Work out the finished part from the listing and answer in its coordinate system (mm). A direction names the side the tool comes from. Round coordinates to 2 decimals unless told otherwise and drop trailing zeros. Loops run counter-clockwise (first coordinate to the right, second up) from the corner with the lowest first, then second, coordinate; pieces in that order, holes last. Notation, with made-up numbers: M 30.25,80 L 35.25,80 A22 cw 35.25,112 Z; hole C 81,-29 d6. An arc over 180 degrees is marked long. One line per item, written item: value.
```python
from build123d import *

# Parameters (mm, degrees)
F0_W     = 4.318
F0_H     = 1.4593527386
F1_DEPTH = 2


with BuildPart() as f1:
    # F0 (on Top) → F1 (new body)
    with BuildSketch(Plane.XY):
        with Locations((4.9730502656, -0.8943877724)):
            Rectangle(F0_W, F0_H)
        with BuildLine():
            Line((7.1320502656, -1.6240641417), (2.8140502656, -1.6240641417))
            Line((2.8140502656, -1.6240641417), (2.8140502656, -0.1647114031))
            Line((2.8140502656, -0.1647114031), (2.6522759268, -0.1647114031))
            Line((2.6522759268, -0.1647114031), (2.6522759268, -19.4612857813))
            Line((2.6522759268, -19.4612857813), (4.8948850305, -19.4612857813))
            Line((4.8948850305, -19.4612857813), (4.8948850305, -11.436884092))
            Line((4.8948850305, -11.436884092), (8.9239793524, -11.436884092))
            Line((8.9239793524, -11.436884092), (13.5950258095, -19.4612857813))
            Line((13.5950258095, -19.4612857813), (16.2473017363, -19.4612857813))
            Line((16.2473017363, -19.4612857813), (11.0061004223, -10.7907085875))
            add(Edge.make_bspline(
                [(14.8873768184, -5.6170811825), (14.8873768184, -9.4434537776), (11.0061004223, -10.7907085875)],
                knots=[0, 0, 0, 1, 1, 1], degree=2))
            add(Edge.make_bspline(
                [(13.1916940404, -1.524636321), (14.8873768184, -2.8845612389), (14.8873768184, -5.6170811825)],
                knots=[0, 0, 0, 1, 1, 1], degree=2))
            add(Edge.make_bspline(
                [(11.4500502656, -0.6254353556), (12.4829894147, -0.9562605066), (13.1916940404, -1.524636321)],
                knots=[0.5820535333, 0.5820535333, 0.5820535333, 1, 1, 1], degree=2))
            Line((11.4500502656, -0.6254353556), (11.4500502656, -1.6240641417))
            Line((11.4500502656, -1.6240641417), (7.1320502656, -1.6240641417))
        make_face()
        with BuildLine():
            Line((7.9737212576, -9.5110276865), (4.8948850305, -9.5110276865))
            Line((4.8948850305, -9.5110276865), (4.8948850305, -2.1328015016))
            Line((4.8948850305, -2.1328015016), (7.8132332238, -2.1328015016))
            add(Edge.make_bspline(
                [(11.436884092, -2.9774753637), (10.3092444862, -2.1328015016), (7.8132332238, -2.1328015016)],
                knots=[0, 0, 0, 1, 1, 1], degree=2))
            add(Edge.make_bspline(
                [(12.5645236978, -5.7353355232), (12.5645236978, -3.8221492257), (11.436884092, -2.9774753637)],
                knots=[0, 0, 0, 1, 1, 1], degree=2))
            add(Edge.make_bspline(
                [(11.4558892539, -8.5671046457), (12.5645236978, -7.6231816049), (12.5645236978, -5.7353355232)],
                knots=[0, 0, 0, 1, 1, 1], degree=2))
            add(Edge.make_bspline(
                [(7.9737212576, -9.5110276865), (10.3472548099, -9.5110276865), (11.4558892539, -8.5671046457)],
                knots=[0, 0, 0, 1, 1, 1], degree=2))
        make_face(mode=Mode.SUBTRACT)
        with BuildLine():
            Line((7.1320502656, -0.1647114031), (7.1320502656, -1.6240641417))
            Line((7.1320502656, -1.6240641417), (11.4500502656, -1.6240641417))
            Line((11.4500502656, -1.6240641417), (11.4500502656, -0.6254353556))
            add(Edge.make_bspline(
                [(7.9441576725, -0.1647114031), (10.0115266043, -0.1647114031), (11.4500502656, -0.6254353556)],
                knots=[0, 0, 0, 0.5820535333, 0.5820535333, 0.5820535333], degree=2))
            Line((7.9441576725, -0.1647114031), (7.1320502656, -0.1647114031))
        make_face()
        Polygon((2.8140502656, 4.8854069319), (2.8140502656, -0.1647114031), (7.1320502656, -0.1647114031), (7.1320502656, 0.4763843317), (4.4037376737, 0.4763843317), (4.4037376737, 2.7849584585), (7.1320502656, 2.7849584585), (7.1320502656, 4.8854069319), align=None)
        with BuildLine():
            Line((7.1320502656, 0.4763843317), (7.1320502656, -0.1647114031))
            Line((7.1320502656, -0.1647114031), (7.9441576725, -0.1647114031))
            add(Edge.make_bspline(
                [(7.9441576725, -0.1647114031), (10.0115266043, -0.1647114031), (11.4500502656, -0.6254353556)],
                knots=[0, 0, 0, 0.5820535333, 0.5820535333, 0.5820535333], degree=2))
            Line((11.4500502656, -0.6254353556), (11.4500502656, 4.8854069319))
            Line((11.4500502656, 4.8854069319), (7.1320502656, 4.8854069319))
            Line((7.1320502656, 4.8854069319), (7.1320502656, 2.7849584585))
            Line((7.1320502656, 2.7849584585), (9.8603628576, 2.7849584585))
            Line((9.8603628576, 2.7849584585), (9.8603628576, 0.4763843317))
            Line((9.8603628576, 0.4763843317), (7.1320502656, 0.4763843317))
        make_face()
    extrude(amount=F1_DEPTH)


solid = f1.part
```
1) For faces 1 (the face through (11.45, 2, 1)), 2 (the face through (7, 2.785, 1)), 3 (the face through (11, -15, 1)), determine the directions among +Z, -Z, +X, -X, +Y, -Y from which every point of the face is accessible in a straight line to the end or side of a thin tool.
Check values:
face 1: +Z, -Z, +X, +Y
face 2: +Z, -Z
face 3: +Z, -Z, -Y
2) Find the intervals of material crossed by probe 1 along Y at (x, z) = (6.5, 1.9); probe 2 along Y at (x, z) = (9, 1.65); probe 3 along X at (y, z) = (-13.5, 1.55), in increasing order. Write a range as from..to.
Check values:
probe 1: -11.44..-9.51, -2.13..0.48, 2.78..4.89
probe 2: -11.57..-9.46, -2.19..0.48, 2.78..4.89
probe 3: 2.65..4.89, 10.12..12.64
3) Each of these flat-tipped pins is pushed along its axis until it touches: pin 1 (0.6 mm diameter, centred on x = 6.5, z = 0.5, fed in from -Y); pin 2 (0.6 mm diameter, centred on y = 2, z = 0.5, fed in from +X); pin 3 (1 mm diameter, centred on y = -14.5, z = 0, fed in from +X). Where does it stop, or does it pass through?
Check values:
pin 1: y = -11.44
pin 2: x = 11.45
pin 3: x = 13.55
4) Find section D-D (y = -17.75). Give the vertices of the cut face in (x, z).
Check values:
outline: M 2.65,0 L 4.89,0 L 4.89,2 L 2.65,2 Z; M 12.6,0 L 15.21,0 L 15.21,2 L 12.6,2 Z
5) Find section B-B (x = 7). Give the vertices of the cut face in (y, z), then the cut area to 3 significant figures.
Check values:
outline: M -11.44,0 L -9.51,0 L -9.51,2 L -11.44,2 Z; M -2.13,0 L 0.48,0 L 0.48,2 L -2.13,2 Z; M 2.78,0 L 4.89,0 L 4.89,2 L 2.78,2 Z
area: 13.3 mm2
6) Find section A-A (y = 1). Give the vertices of the cut face in (x, z), then the cut area to 3 significant figures.
Check values:
outline: M 2.81,0 L 4.4,0 L 4.4,2 L 2.81,2 Z; M 9.86,0 L 11.45,0 L 11.45,2 L 9.86,2 Z
area: 6.36 mm2
7) Find section C-C (z = 0.95). Give the number of separate pieces and of enclosed holes in the cut face, then the cut area to 3 significant figures.
Check values:
separate pieces: 1
enclosed holes: 2
area: 143 mm2
8) The mould has two halves that part along X. Classify faces 4 (the face through (13.663, -15.187, 0.986)), 5 (the face through (4.404, 2, 1)), 6 (the face through (7, 4.885, 1)), 7 (the face through (2.652, -10, 1)): +X half, -X half, draft (parallel to the pull), parting line (faces both ways), or undercut.
Check values:
face 4: +X half
face 5: undercut
face 6: draft
face 7: -X half
